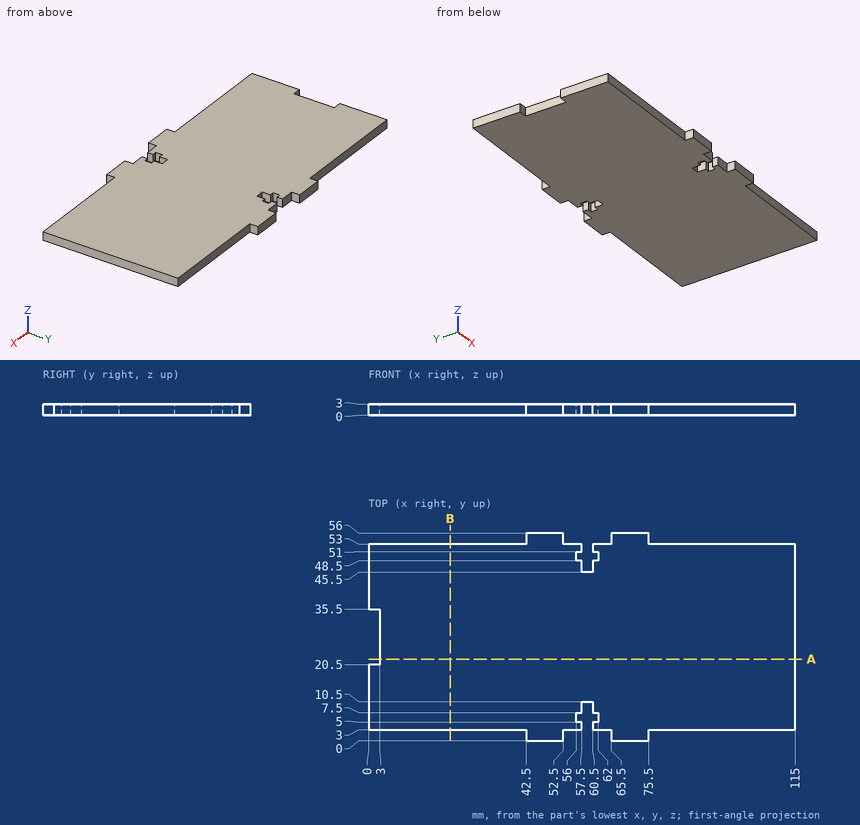
The drawing under review shows one solid part. Ordinate dimensions are in mm from its lowest x, y, z. Round coordinates to 2 decimals unless told otherwise and drop trailing zeros. Write each loop counter-clockwise with the first axis right and the second up, starting at its lowest first coordinate (ties: lowest second). Pieces come first, ordered by that corner, then holes.
(1) We need section B-B on x = 22. Give the boundary of the cut face in (y, z).
(2) We need section A-A on y = 22. Give the boundary of the cut face in (x, z).
(3) Wall thickness on L1, parallel to X at y = 2, z = 1.7; L2, parallel to X at y = 47, z = 0.9; L3, parallel to X at y = 24, z = 0.7: over which ranges is each line inside the solid? List them lowest first.
(4) Insertion check: pin 1 (0.9 mm diameter, centred on y = 47, z = 1.5, fed in from -X); pin 2 (0.9 mm diameter, centred on y = 1.5, z = 2, fed in from +X); pin 3 (0.9 mm diameter, centred on x = 63.5, z = 1, fed in from +Y); pin 4 (1.6 mm diameter, centred on x = 61.5, z = 1, fed in from -Y). Each pin has a flat end and moves straight along its axis. Give the tip position at first contact, or say it passes through.
Findings below:
1. outline: (3, 0) - (53, 0) - (53, 3) - (3, 3) - close
2. outline: (3, 0) - (115, 0) - (115, 3) - (3, 3) - close
3. L1: x = 42.5 to 52.5, 65.5 to 75.5
3. L2: x = 0 to 57.5, 60.5 to 115
3. L3: x = 3 to 115
4. pin 1: stops at x = 0
4. pin 2: stops at x = 75.5
4. pin 3: stops at y = 53
4. pin 4: stops at y = 3
